Design review of the part built by this model. Coordinates are the model's own, in mm. Face numbers are marked on the shaded views. Round coordinates to 2 decimals unless told otherwise and drop trailing zeros. Loops run counter-clockwise (first coordinate to the right, second up) from the corner with the lowest first, then second, coordinate; pieces in that order, holes last. Notation, with made-up numbers: (10.25, 45) - (43.25, 45) arc R35 cw to (43.25, 83) - close; hole circle Ø8 at (32.5, -10). An arc over 180 degrees is marked (long way). Return JSON: item names as keys, results as strings. Group by question number.
(1) Wall thickness on L1, parallel to X at y = 9, z = -13.5; L2, parallel to Z at x = 43, y = -7.5; L3, parallel to Y at x = 59.7, z = -10: over which ranges is each line inside the solid? List them lowest first. Write a range as [from, to].
(2) Clearance check with flat-ended pins moving along their axes: pin 1 (7 mm diameter, centred on y = 15.86, z = -30, fed in from +X); pin 2 (1.1 mm diameter, centred on x = 0.5, y = -25.5, fed in from -Z); pin 3 (0.8 mm diameter, centred on x = 59.5, y = -24, fed in from +Z). State where each tip first meets the part, or that it passes through.
(3) We need section C-C, the plane y = -11.5. Write out the cut boundary in (x, z).
(4) We need section D-D, the plane x = 18. Write out the cut boundary in (y, z), and give its area (3 significant figures).
(5) The part is to be moulded in two halves that separate along X. For the marked faces 1, 2, 3 and 4, say which applies: pulls with the +X half, pulls with the -X half, needs draft (parallel to the pull), parting line crosses it, or undercut.
(6) We need section B-B, the plane z = -5. Write out the cut boundary in (x, y), and give its area (3 significant figures).
(7) We need section A-A, the plane z = -10. Write out the cut boundary in (x, y), and give its area (3 significant figures).
from build123d import *

# Parameters (mm, degrees)
SKETCH1_R           = 1.5
BOSS_EXTRUDE1_DEPTH = 1
BOSS_EXTRUDE2_START = -1
SKETCH2_W           = 1
SKETCH2_H           = 15
BOSS_EXTRUDE2_DEPTH = 30
FILLET1_R           = 1
CUT_EXTRUDE1_REACH  = 62
SKETCH3_R           = 4


with BuildPart() as part:
    # Sketch1 → Boss-Extrude1 (new body)
    with BuildSketch(Plane(origin=(0, 0, 0), x_dir=(0, 0, -1), z_dir=(1, 0, 0))):
        with BuildLine():
            Line((0, 0), (22.928644487, 22.928644487))
            ThreePointArc((22.928644487, 22.928644487), (37.07078011, 22.928644487), (37.07078011, 8.786508863))
            Line((37.07078011, 8.786508863), (20, -8.284271247))
            Line((20, -8.284271247), (20, -38.019))
            ThreePointArc((20, -38.019), (10, -48.019), (0, -38.019))
            Line((0, -38.019), (0, 0))
        make_face()
        with Locations((29.999712299, 15.857576675)):
            Circle(SKETCH1_R, mode=Mode.SUBTRACT)
        with Locations((10, -38.019)):
            Circle(SKETCH1_R, mode=Mode.SUBTRACT)
    boss_extrude1 = extrude(amount=BOSS_EXTRUDE1_DEPTH)

    # Sketch2 → Boss-Extrude2 (add)
    with BuildSketch(Plane(origin=(1, 0, 0), x_dir=(0, 0, -1), z_dir=(1, 0, 0)).offset(BOSS_EXTRUDE2_START)):
        with Locations((-0.5, -7.5)):
            Rectangle(SKETCH2_W, SKETCH2_H)
    boss_extrude2 = extrude(amount=BOSS_EXTRUDE2_DEPTH)

    # Mirror2: Boss-Extrude1, Boss-Extrude2 across plane
    add(boss_extrude1.mirror(Plane.ZY.offset(-30)))
    add(boss_extrude2.mirror(Plane.ZY.offset(-30)))

    # Fillet1
    fillet1_edges = [part.edges().sort_by_distance(p)[0] for p in [
        (1, -7.5, 0),
        (59, -7.5, 0),
        (0, -7.5, 1),
        (60, -7.5, 1),
    ]]
    fillet(fillet1_edges, radius=FILLET1_R)

    # Sketch3 → Cut-Extrude1 (cut, up to next)
    with BuildSketch(Plane(origin=(60, 0, 0), x_dir=(0, 0, -1), z_dir=(1, 0, 0)), mode=Mode.PRIVATE) as cut_extrude1_sk1:
        with Locations((29.999712299, 15.857576675)):
            Circle(SKETCH3_R)
    cut_extrude1_tool1 = extrude(cut_extrude1_sk1.sketch, amount=-CUT_EXTRUDE1_REACH, mode=Mode.PRIVATE) & part.part
    add(cut_extrude1_tool1.solids().sort_by_distance((60, 15.857577, -29.999712))[0], mode=Mode.SUBTRACT)
    # Sketch3 → Cut-Extrude1 (cut, up to next)
    with BuildSketch(Plane(origin=(60, 0, 0), x_dir=(0, 0, -1), z_dir=(1, 0, 0)), mode=Mode.PRIVATE) as cut_extrude1_sk2:
        with Locations((10, -38.019)):
            Circle(SKETCH3_R)
    cut_extrude1_tool2 = extrude(cut_extrude1_sk2.sketch, amount=-CUT_EXTRUDE1_REACH, mode=Mode.PRIVATE) & part.part
    add(cut_extrude1_tool2.solids().sort_by_distance((60, -38.019, -10))[0], mode=Mode.SUBTRACT)


solid = part.part
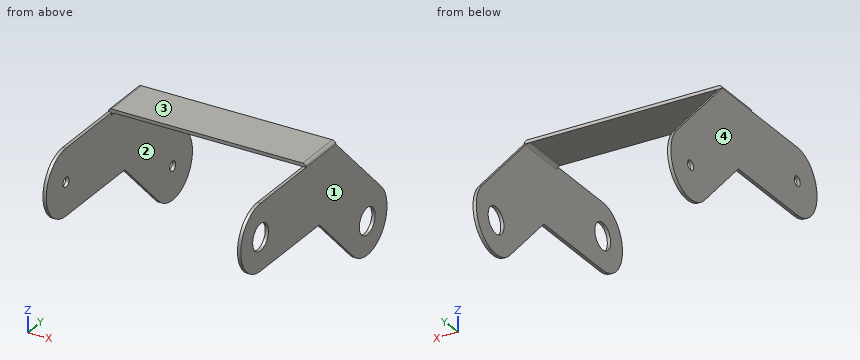
Solutions:
{
 "1": {"L1": "[0, 1], [59, 60]", "L2": "[0, 1]", "L3": "[-48.02, -42.02], [-34.02, 10]"},
 "2": {"pin 1": "x = 1", "pin 2": "z = -20", "pin 3": "z = 0"},
 "3": {"outline": "(0, -20) - (1, -20) - (1, -1) arc R1 cw to (2, 0) - (58, 0) arc R1 cw to (59, -1) - (59, -20) - (60, -20) - (60, 0) arc R1 ccw to (59, 1) - (1, 1) arc R1 ccw to (0, 0) - close"},
 "4": {"outline": "(-15, 0) - (0, 0) - (0, 1) - (-15, 1) - close", "area": "15.0 mm^2"},
 "5": {"face 1": "pulls with the +X half", "face 2": "undercut", "face 3": "needs draft", "face 4": "pulls with the -X half"},
 "6": {"outline": "(0, -46.68) - (1, -46.68) - (1, 5) - (0, 5) - close; (59, -46.68) - (60, -46.68) - (60, 5) - (59, 5) - close", "area": "103 mm^2"},
 "7": {"outline": "(0, -48.02) - (1, -48.02) - (1, -39.52) - (0, -39.52) - close; (0, -36.52) - (1, -36.52) - (1, 10) - (0, 10) - close; (59, -48.02) - (60, -48.02) - (60, -42.02) - (59, -42.02) - close; (59, -34.02) - (60, -34.02) - (60, 10) - (59, 10) - close", "area": "105 mm^2"}
}
